Build history of the part. All positions in model axes, mm. Give positions to 0.01 mm unless a question says otherwise; leave off trailing zeros. Order: outer loops, then holes, each group sorted by start corner. A loop starts at its lowest first (then second) coordinate and runs counter-clockwise, first axis right, second up. Notation, with made-up numbers: (17, -38.5) -> (63, -38.5) arc R20 cw to (63, -6.5) -> close; hole circle Ø1 at (-17, 35). An arc over 180 degrees is marked (long way). Use a Markdown table: item, result. Add a question column.
```python
from build123d import *

# Parameters (mm, degrees)
SKETCH_R        = 95
PAD_DEPTH       = 3
SKETCH001_R     = 1.25
POCKET_DEPTH    = 3.001
SKETCH002_R     = 1.75
SKETCH002_W     = 16
SKETCH002_H     = 55
POCKET001_DEPTH = 540.435647
SKETCH003_R     = 1.75
POCKET002_DEPTH = 3.001
SKETCH004_R     = 1
POCKET003_DEPTH = 3.001


with BuildPart() as part:
    # Sketch → Pad (new body)
    with BuildSketch(Plane.XY):
        Circle(SKETCH_R)
    extrude(amount=PAD_DEPTH)

    # Sketch001 (on Face3 of Pad) → Pocket (cut, through all)
    with BuildSketch(Plane.XY.offset(3)):
        with Locations((-15, 71)):
            Circle(SKETCH001_R)
        with Locations((15, 71)):
            Circle(SKETCH001_R)
        with Locations((15, 47)):
            Circle(SKETCH001_R)
        with Locations((-15, 47)):
            Circle(SKETCH001_R)
    extrude(amount=-POCKET_DEPTH, mode=Mode.SUBTRACT)

    # Sketch002 (on Face3 of Pocket) → Pocket001 (cut, through all)
    with BuildSketch(Plane.XY.offset(3)):
        with Locations((-66, -11)):
            Circle(SKETCH002_R)
        with Locations((-42, -11)):
            Circle(SKETCH002_R)
        with Locations((-66, -41)):
            Circle(SKETCH002_R)
        with Locations((-42, -41)):
            Circle(SKETCH002_R)
        with Locations((-88, -26)):
            Rectangle(SKETCH002_W, SKETCH002_H)
    pocket001 = extrude(amount=-POCKET001_DEPTH, mode=Mode.SUBTRACT)

    # Mirrored: Pocket001 across YZ
    add(pocket001.mirror(Plane.YZ), mode=Mode.SUBTRACT)

    # Sketch003 (on Face4 of Mirrored) → Pocket002 (cut, through all)
    with BuildSketch(Plane.XY.offset(3)):
        with Locations((-36, 79.202273)):
            Circle(SKETCH003_R)
        with Locations((36, 79.202273)):
            Circle(SKETCH003_R)
        with Locations((-71, -50.27922)):
            Circle(SKETCH003_R)
        with Locations((71, -50.27922)):
            Circle(SKETCH003_R)
        with Locations((-86, 13.152946)):
            Circle(SKETCH003_R)
        with Locations((86, 13.152946)):
            Circle(SKETCH003_R)
        with Locations((0, -87)):
            Circle(SKETCH003_R)
    extrude(amount=-POCKET002_DEPTH, mode=Mode.SUBTRACT)

    # Sketch004 (on Face4 of Pocket002) → Pocket003 (cut, through all)
    with BuildSketch(Plane.XY.offset(3)):
        with Locations((-62.5, -4)):
            Circle(SKETCH004_R)
        with Locations((-62.5, 54)):
            Circle(SKETCH004_R)
        with Locations((-13.5, 54)):
            Circle(SKETCH004_R)
        with Locations((-13.5, -4)):
            Circle(SKETCH004_R)
        with Locations((22.2, 52.5)):
            Circle(SKETCH004_R)
        with Locations((7, 1.7)):
            Circle(SKETCH004_R)
        with Locations((55.2, 0.4)):
            Circle(SKETCH004_R)
        with Locations((50.1, 52.5)):
            Circle(SKETCH004_R)
        with BuildLine():
            ThreePointArc((-10, -40), (-14, -44), (-10, -48))
            Line((-10, -48), (10, -48))
            ThreePointArc((10, -48), (14, -44), (10, -40))
            Line((-10, -40), (10, -40))
        make_face()
    extrude(amount=-POCKET003_DEPTH, mode=Mode.SUBTRACT)


solid = part.part
```
(1) Band-saw the part on A-A on y = -29. Give the cut face in (x, z).
(2) Band-saw the part on B-B on x = -46. Give the cut face in (y, z), plus the area to 3 significant figures.
(3) Pin check, flat tip, straight feed: pin 1 Ø1.5 at (x, z) = (-62, 2.5) entering from -Y. Stop position of the tip, or through.
(4) Band-saw the part on C-C on z = 0.55. State how many separate pieces and enclosed holes the cut face has, plus the area to 3 significant figures.
(5) Wall check: probe 1 along Y at (x, z) = (-40.5, 2.55); probe 2 along Y at (x, z) = (-13.5, 1.9); probe 3 along Y at (x, z) = (-66.5, 2.1). Give the ranges that are in metal, low to high.
Response:
| question | item | result |
|---|---|---|
| 1 | outline | (-80, 0) -> (80, 0) -> (80, 3) -> (-80, 3) -> close |
| 2 | outline | (-83.12, 0) -> (83.12, 0) -> (83.12, 3) -> (-83.12, 3) -> close |
| 2 | area | 499 mm² |
| 3 | pin 1 | stops at y = -72.62 |
| 4 | separate pieces | 1 |
| 4 | enclosed holes | 28 |
| 4 | area | 26,900 mm² |
| 5 | probe 1 | y = -85.93 to -41.9, -40.1 to -11.9, -10.1 to 85.93 |
| 5 | probe 2 | y = -94.04 to -45.94, -42.06 to -5, -3 to 53, 55 to 94.04 |
| 5 | probe 3 | y = -67.84 to -42.68, -39.32 to -12.68, -9.32 to 67.84 |
